Read the model definition and answer for the solid it produces. Units are mm, in the model's axes. Face numbers are marked on the shaded views. A direction names the side the tool comes from. Coordinates: 2 decimals unless noted, no trailing zeros. Order: outer loops, then holes, each group sorted by start corner. A loop starts at its lowest first (then second) coordinate and runs counter-clockwise, first axis right, second up. Notation, with made-up numbers: (-31, -12.75) -> (21, -12.75) arc R34 ccw to (21, 25.25) -> close; hole circle Ø2 at (7, 54.25). An arc over 180 degrees is marked (long way). Answer as a JSON object with one key per item and string values. Group by question number.
1) Consider L1, parallel to Y at x = -2.5, z = -24; L2, parallel to Y at x = 3.25, z = -24; L3, parallel to Y at x = 2.5, z = -44. Determine where each line is inside the solid, lowest interval first.
2) Section C-C on z = -44.5 is taken. Determine the outline of the cut face in (x, y), and give its area (3 significant figures).
3) Section A-A on x = -4 is taken. Count the separate pieces of the cut face and the enclosed holes in it, and give its area (3 significant figures).
4) A tool of negligible diameter and unlimited length cuts with its end or side. For the marked faces 1, 2 and 3, from which of +Z, -Z, +X, -X, +Y, -Y can it reach the whole face along a straight path? Write none if from no direction.
5) Given pin 1 (4 mm diameter, centred on y = 7.5, z = -33, fed in from -X); pin 2 (1 mm diameter, centred on y = -22, z = -17, fed in from +X); pin 3 (12 mm diameter, centred on x = -4.5, y = -54.5, fed in from -Z); pin 4 (3 mm diameter, centred on y = -36, z = -16, fed in from -X), each flat-ended and moving along its own axis, determine where each tip first touches the part or whether it passes through.
from build123d import *

# Parameters (mm, degrees)
SKETCH1_W           = 48
SKETCH1_H           = 48
BOSS_EXTRUDE1_DEPTH = 75
SKETCH2_W           = 48
SKETCH2_H           = 48
BOSS_EXTRUDE2_DEPTH = 7.5
FILLET1_R           = 24
SKETCH3_R           = 5
CUT_EXTRUDE1_DEPTH  = 15
SKETCH4_R           = 5
BOSS_EXTRUDE3_DEPTH = 7.5


with BuildPart() as part:
    # Sketch1 → Boss-Extrude1 (new, symmetric)
    with BuildSketch(Plane(origin=(0, 0, 0), x_dir=(1, 0, 0), z_dir=(0, 1, 0))):
        with Locations((24, 24)):
            Rectangle(SKETCH1_W, SKETCH1_H)
    extrude(amount=BOSS_EXTRUDE1_DEPTH, both=True)

    # Sketch2 → Boss-Extrude2 (add, symmetric)
    with BuildSketch(Plane.ZY):
        with Locations((-24, 51)):
            Rectangle(SKETCH2_W, SKETCH2_H)
        with Locations((-24, -51)):
            Rectangle(SKETCH2_W, SKETCH2_H)
    extrude(amount=BOSS_EXTRUDE2_DEPTH, both=True)

    # Fillet1
    fillet1_edges = [part.edges().sort_by_distance(p)[0] for p in [
        (48, 75, -24),
        (0, 0, -48),
        (20.25, 75, -48),
        (0, 0, 0),
        (-3.75, 27, -48),
        (-3.75, 27, 0),
        (-3.75, -27, 0),
        (-3.75, -27, -48),
        (20.25, -75, -48),
        (48, -75, -24),
        (20.25, -75, 0),
        (48, 0, -48),
        (48, 0, 0),
        (20.25, 75, 0),
    ]]
    fillet(fillet1_edges, radius=FILLET1_R - 0.0001)  # a hair under: the kernel refuses the full size

    # Sketch3 → Cut-Extrude1 (cut)
    with BuildSketch(Plane.ZY.offset(7.5)):
        with Locations((-24, -51)):
            Circle(SKETCH3_R)
    extrude(amount=-CUT_EXTRUDE1_DEPTH, mode=Mode.SUBTRACT)

    # Sketch4 → Boss-Extrude3 (add, symmetric)
    with BuildSketch(Plane.ZY.offset(7.5)):
        with Locations((-24, 51)):
            Circle(SKETCH4_R)
    extrude(amount=BOSS_EXTRUDE3_DEPTH, both=True)


solid = part.part
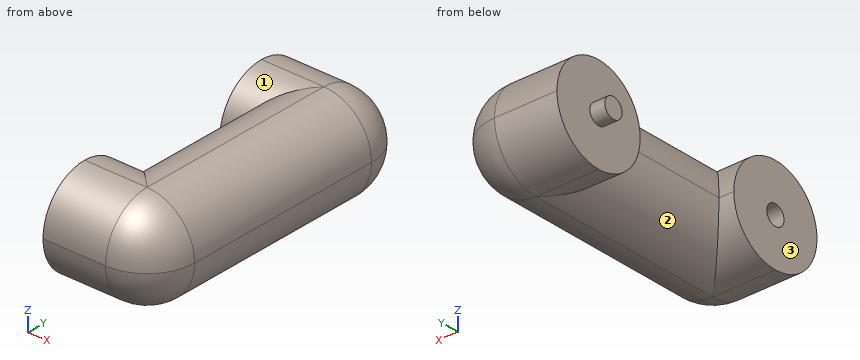
Worked answers:
{
 "1": {"L1": "y = -75 to -56, -46 to -27, 27 to 75", "L2": "y = -75 to -56, -46 to 75", "L3": "y = -64.27 to -37.73, 37.73 to 64.27"},
 "2": {"outline": "(-7.5, -63.48) -> (24, -63.48) arc R12.48 ccw to (36.48, -51) -> (36.48, 51) arc R12.48 ccw to (24, 63.48) -> (-7.5, 63.48) -> (-7.5, 38.52) -> (11.52, 38.52) -> (11.52, -38.52) -> (-7.5, -38.52) -> close", "area": "4,050 mm²"},
 "3": {"separate pieces": "2", "enclosed holes": "1", "area": "3,540 mm²"},
 "4": {"face 1": "+Z, -X", "face 2": "-Z, -X", "face 3": "+Z, -Z, -X, -Y"},
 "5": {"pin 1": "stops at x = 1.04", "pin 2": "stops at x = 47.1", "pin 3": "stops at z = -48", "pin 4": "stops at x = -7.5"}
}
